```python
from build123d import *

# Parameters (mm, degrees)
SKETCH_1_W                 = 34
SKETCH_1_H                 = 36
EXTRUDE_1_DEPTH            = 10
SHELL_1_T                  = -1
SHELL_1_THICKNESS_2_FACE_W = 34
SHELL_1_THICKNESS_2_FACE_H = 32
SHELL_1_THICKNESS_2_DEPTH  = 1
CUT_EXTRUDE_START          = 8
SKETCH_2_W                 = 12.58
SKETCH_2_H                 = 6.98
CUT_EXTRUDE_1_DEPTH        = 5.0005
SKETCH_6_W                 = 14.7
SKETCH_6_H                 = 11.8
CUT_EXTRUDE_2_DEPTH        = 1
FILLET_2_R                 = 0.5
CUT_EXTRUDE_START_2        = 10
CUT_EXTRUDE_3_DEPTH        = 2
CUT_EXTRUDE_START_3        = -16
CUT_EXTRUDE_4_DEPTH        = 1
CUT_EXTRUDE_START_4        = 17
SKETCH_13_W                = 9.193413451
SKETCH_13_H                = 1.5
CUT_EXTRUDE_5_DEPTH        = 0.5


with BuildPart() as part:
    # 草图1 → 凸台-拉伸1 (new body)
    with BuildSketch(Plane(origin=(0, 0, 0), x_dir=(1, 0, 0), z_dir=(0, 1, 0))):
        Rectangle(SKETCH_1_W, SKETCH_1_H)
    extrude(amount=EXTRUDE_1_DEPTH)

    # 抽壳1
    shell_1_openings = [part.faces().sort_by_distance(p)[0] for p in [
        (0, 0, 0),
    ]]
    offset(amount=SHELL_1_T, openings=shell_1_openings, kind=Kind.INTERSECTION)

    # 抽壳1 thickness 2 face (on inner face of the shell) → 抽壳1 thickness 2 (add)
    with BuildSketch(Plane.ZX.offset(9)):
        Rectangle(SHELL_1_THICKNESS_2_FACE_W, SHELL_1_THICKNESS_2_FACE_H)
    extrude(amount=-SHELL_1_THICKNESS_2_DEPTH)

    # 草图2 → 切除-拉伸1 (cut, symmetric)
    with BuildSketch(Plane(origin=(0, 0, 0), x_dir=(1, 0, 0), z_dir=(0, 1, 0)).offset(CUT_EXTRUDE_START)):
        with Locations((0.114253814, 10.274424553)):
            Rectangle(SKETCH_2_W, SKETCH_2_H)
    extrude(amount=CUT_EXTRUDE_1_DEPTH, both=True, mode=Mode.SUBTRACT)

    # 草图6 → 切除-拉伸2 (cut, symmetric)
    with BuildSketch(Plane(origin=(0, 0, 0), x_dir=(1, 0, 0), z_dir=(0, 1, 0)).offset(CUT_EXTRUDE_START)):
        with Locations((0.212081247, 8.751285152)):
            Rectangle(SKETCH_6_W, SKETCH_6_H)
    extrude(amount=CUT_EXTRUDE_2_DEPTH, both=True, mode=Mode.SUBTRACT)

    # 圆角2
    fillet_2_edges = [part.edges().sort_by_distance(p)[0] for p in [
        (6.404253814, 10, -10.274424553),
        (0.114253814, 10, -6.784424553),
        (-6.175746186, 10, -10.274424553),
        (0.114253814, 10, -13.764424553),
    ]]
    fillet(fillet_2_edges, radius=FILLET_2_R)

    # 草图10 → 切除-拉伸3 (cut)
    with BuildSketch(Plane(origin=(0, 0, 0), x_dir=(1, 0, 0), z_dir=(0, 1, 0)).offset(CUT_EXTRUDE_START_2)):
        with BuildLine():
            Line((-3.993743906, -1.215281594), (-2.463768403, -2.690446502))
            ThreePointArc((-2.463768403, -2.690446502), (1.744606129, -2.322550765), (4.505547025, -5.519888538))
            Line((4.505547025, -5.519888538), (6.628721392, -5.515926654))
            ThreePointArc((6.628721392, -5.515926654), (2.52183734, -0.390898934), (-3.993743906, -1.215281594))
        make_face()
        with BuildLine():
            Line((-5.750245846, -3.142252551), (-4.035268841, -4.309111683))
            ThreePointArc((-4.035268841, -4.309111683), (-4.509884123, -7.752654512), (-2.464252289, -10.56310595))
            Line((-2.464252289, -10.56310595), (-3.477509556, -12.370007953))
            ThreePointArc((-3.477509556, -12.370007953), (-6.52500842, -8.22682935), (-5.750245846, -3.142252551))
        make_face()
        with BuildLine():
            Line((-0.33755867, -11.264535632), (-0.979652593, -13.267970949))
            ThreePointArc((-0.979652593, -13.267970949), (3.836702752, -12.136836694), (6.57348953, -8.015339194))
            Line((6.57348953, -8.015339194), (4.50812982, -7.787936955))
            ThreePointArc((4.50812982, -7.787936955), (2.714792905, -10.403644562), (-0.33755867, -11.264535632))
        make_face()
    extrude(amount=-CUT_EXTRUDE_3_DEPTH, mode=Mode.SUBTRACT)

    # 草图11 → 切除-拉伸4 (cut)
    with BuildSketch(Plane(origin=(0, 0, 0), x_dir=(0, 0, -1), z_dir=(1, 0, 0)).offset(CUT_EXTRUDE_START_3)):
        with BuildLine():
            Line((13.165354419, 7.763482474), (12.615354419, 7.763482474))
            ThreePointArc((12.615354419, 7.763482474), (12.261801028, 7.617035865), (12.115354419, 7.263482474))
            Line((12.115354419, 7.263482474), (12.115354419, 2.663482474))
            ThreePointArc((12.115354419, 2.663482474), (12.261801028, 2.309929083), (12.615354419, 2.163482474))
            Line((12.615354419, 2.163482474), (13.165354419, 2.163482474))
            ThreePointArc((13.165354419, 2.163482474), (13.518907809, 2.309929083), (13.665354419, 2.663482474))
            Line((13.665354419, 2.663482474), (13.665354419, 7.263482474))
            ThreePointArc((13.665354419, 7.263482474), (13.518907809, 7.617035865), (13.165354419, 7.763482474))
        make_face()
        with BuildLine():
            Line((15.855458394, 7.745816392), (15.305458394, 7.745816392))
            ThreePointArc((15.305458394, 7.745816392), (14.951905004, 7.599369782), (14.805458394, 7.245816392))
            Line((14.805458394, 7.245816392), (14.805458394, 2.645816392))
            ThreePointArc((14.805458394, 2.645816392), (14.951905004, 2.292263001), (15.305458394, 2.145816392))
            Line((15.305458394, 2.145816392), (15.855458394, 2.145816392))
            ThreePointArc((15.855458394, 2.145816392), (16.209011785, 2.292263001), (16.355458394, 2.645816392))
            Line((16.355458394, 2.645816392), (16.355458394, 7.245816392))
            ThreePointArc((16.355458394, 7.245816392), (16.209011785, 7.599369782), (15.855458394, 7.745816392))
        make_face()
        with BuildLine():
            Line((10.524610149, 7.763448499), (9.974610149, 7.763448499))
            ThreePointArc((9.974610149, 7.763448499), (9.621056758, 7.617001889), (9.474610149, 7.263448499))
            Line((9.474610149, 7.263448499), (9.474610149, 2.663448499))
            ThreePointArc((9.474610149, 2.663448499), (9.621056758, 2.309895108), (9.974610149, 2.163448499))
            Line((9.974610149, 2.163448499), (10.524610149, 2.163448499))
            ThreePointArc((10.524610149, 2.163448499), (10.878163539, 2.309895108), (11.024610149, 2.663448499))
            Line((11.024610149, 2.663448499), (11.024610149, 7.263448499))
            ThreePointArc((11.024610149, 7.263448499), (10.878163539, 7.617001889), (10.524610149, 7.763448499))
        make_face()
    extrude(amount=-CUT_EXTRUDE_4_DEPTH, mode=Mode.SUBTRACT)

    # 草图13 → 切除-拉伸5 (cut)
    with BuildSketch(Plane.XY.offset(CUT_EXTRUDE_START_4)):
        with Locations((9.633284571, 0.749986932)):
            Rectangle(SKETCH_13_W, SKETCH_13_H)
    extrude(amount=CUT_EXTRUDE_5_DEPTH, mode=Mode.SUBTRACT)


solid = part.part
```
Verification items for the finished model (mm, model axes). A direction names the side the tool comes from. Coordinates: 2 decimals unless noted, no trailing zeros. Loops run counter-clockwise (first coordinate to the right, second up) from the corner with the lowest first, then second, coordinate; pieces in that order, holes last. Notation, with made-up numbers: (-6.5, 86) - (24.5, 86) arc R13 cw to (24.5, 110) - close; hole circle Ø4 at (76, -6.5). An arc over 180 degrees is marked (long way). Return JSON: item names as keys, results as strings.
1. Section check C-C, the plane x = 6. Record the boundary of the cut face in (y, z).
Established:
{"outline": "(0, -18) - (10, -18) - (10, -14.26) arc R0.5 ccw to (9.5, -13.76) - (9, -13.76) - (9, -14.65) - (8, -14.65) - (8, -17) - (0, -17) - close; (0, 17.5) - (1.5, 17.5) - (1.5, 17) - (8, 17) - (8, 9.65) - (10, 9.65) - (10, 18) - (0, 18) - close; (8, -2.85) - (9, -2.85) - (9, -6.78) - (9.5, -6.78) arc R0.5 ccw to (10, -6.28) - (10, 3.59) - (8, 3.59) - close; (8, 5.52) - (10, 5.52) - (10, 7.95) - (8, 7.95) - close"}
2. Section check D-D, the plane x = 11. Record the boundary of the cut face in (y, z), then the cut area to 4 significant figures.
Established:
{"outline": "(0, -18) - (10, -18) - (10, 18) - (0, 18) - (0, 17.5) - (1.5, 17.5) - (1.5, 17) - (8, 17) - (8, -17) - (0, -17) - close", "area": "87.25 mm2"}
3. Thickness scan on L1, parallel to Z at x = 9, y = 3.25; L2, parallel to X at y = 0.75, z = -11; L3, parallel to X at y = 8.5, z = 4. Record the ranges inside material, lowest first.
Established:
{"L1": "z = -18 to -17, 17 to 18", "L2": "x = -17 to -16, 16 to 17", "L3": "x = -17 to -6.19, -4.49 to 3.83, 6.19 to 17"}
4. Section check A-A, the plane y = 6. Record the boundary of the cut face in (x, z).
Established:
{"outline": "(-17, -18) - (17, -18) - (17, 18) - (-17, 18) - (-17, -9.47) - (-16, -9.47) - (-16, 17) - (16, 17) - (16, -17) - (-16, -17) - (-16, -16.36) - (-17, -16.36) - close; (-17, -14.81) - (-16, -14.81) - (-16, -13.67) - (-17, -13.67) - close; (-17, -12.12) - (-16, -12.12) - (-16, -11.02) - (-17, -11.02) - close"}
5. Mould release check, pull along Y, two halves, no side actions. Record for faces 5 (the flat face through (-16.5, 4.9, -11.025)), 6 (the flat face through (0, 9, -6)), 7 (the cylindrical face through (2.75, 9.01, 10.38)): +Y half, -Y half, draft (parallel to the pull), parting line (faces both ways), or undercut.
Established:
{"face 5": "undercut", "face 6": "-Y half", "face 7": "draft"}
6. Section check B-B, the plane x = -10. Record the boundary of the cut face in (y, z).
Established:
{"outline": "(0, -18) - (10, -18) - (10, 18) - (0, 18) - (0, 17) - (8, 17) - (8, -17) - (0, -17) - close"}
7. Go/stop test with flat-tipped pins: pin 1 (9.5 mm diameter, centred on x = -3, z = -11.5, fed in from -Y); pin 2 (6 mm diameter, centred on x = 4, z = -10, fed in from +Y). Record where each tip stops, or that it passes through.
Established:
{"pin 1": "stops at y = 8", "pin 2": "stops at y = 10"}
8. Tool access check on faces 1 (the cylindrical face through (-4.522, 9.014, 7.704)), 2 (the flat face through (-16.5, 4.9, -13.665)), 3 (the flat face through (-0.2, 10, -0.3)), 4 (the flat face through (16, 4, 0)). Record the directions out of +Z, -Z, +X, -X, +Y, -Y that give a thin tool (end or side, any length) a straight path to the whole face; none if there is none.
Established:
{"face 1": "+Y, -Y", "face 2": "-X", "face 3": "+Z, -Z, +X, -X, +Y", "face 4": "-Y"}
